```python
from build123d import *

# Parameters (mm, degrees)
SKETCH1_R           = 27
SKETCH1_R_2         = 14
BOSS_EXTRUDE1_DEPTH = 10
SKETCH2_R           = 32.5
BOSS_EXTRUDE2_DEPTH = 2
SKETCH3_W           = 5
SKETCH3_H           = 4.39677325
SKETCH3_W_2         = 4.39677325
SKETCH3_H_2         = 5
BOSS_EXTRUDE3_DEPTH = 10
CUT_EXTRUDE1_REACH  = 49.503
SKETCH4_R           = 0.9
BOSS_EXTRUDE4_DEPTH = 10
BOSS_EXTRUDE5_START = -2
SKETCH6_R           = 14
BOSS_EXTRUDE5_DEPTH = 2


with BuildPart() as part:
    # Sketch1 → Boss-Extrude1 (new body)
    with BuildSketch(Plane(origin=(0, 0, 0), x_dir=(1, 0, 0), z_dir=(0, 1, 0))):
        with Locations(Location((0, 0, 0), (0, 0, 270))):
            Circle(SKETCH1_R)
        with Locations(Location((0, 0, 0), (0, 0, 270))):
            Circle(SKETCH1_R_2, mode=Mode.SUBTRACT)
        with BuildLine():
            Line((-17.5, -17.853571071), (-11.2, -11.426285486))
            ThreePointArc((-11.2, -11.426285486), (0, 16), (11.2, -11.426285486))
            Line((11.2, -11.426285486), (17.5, -17.853571071))
            ThreePointArc((17.5, -17.853571071), (0, 25), (-17.5, -17.853571071))
        make_face(mode=Mode.SUBTRACT)
    extrude(amount=BOSS_EXTRUDE1_DEPTH)

    # Sketch2 → Boss-Extrude2 (add)
    with BuildSketch(Plane.XZ):
        with Locations(Location((0, 0, 0), (0, 0, 270))):
            Circle(SKETCH2_R)
    extrude(amount=BOSS_EXTRUDE2_DEPTH)

    # Sketch3 → Boss-Extrude3 (add)
    with BuildSketch(Plane(origin=(0, 0, 0), x_dir=(1, 0, 0), z_dir=(0, 1, 0))):
        with Locations((0, 27.601613375)):
            Rectangle(SKETCH3_W, SKETCH3_H)
        with Locations((27.601613375, 0)):
            Rectangle(SKETCH3_W_2, SKETCH3_H_2)
        with Locations((0, -27.601613375)):
            Rectangle(SKETCH3_W, SKETCH3_H)
        with Locations((-27.601613375, 0)):
            Rectangle(SKETCH3_W_2, SKETCH3_H_2)
    extrude(amount=BOSS_EXTRUDE3_DEPTH)

    # Sketch4 → Cut-Extrude1 (cut, up to next)
    with BuildSketch(Plane.XZ.offset(2), mode=Mode.PRIVATE) as cut_extrude1_sk1:
        with Locations(Location((0, -7, 0), (0, 0, 270))):
            Circle(SKETCH4_R)
    cut_extrude1_tool1 = extrude(cut_extrude1_sk1.sketch, amount=-CUT_EXTRUDE1_REACH, mode=Mode.PRIVATE) & part.part
    # Sketch4 → Cut-Extrude1 (cut, up to next)
    with BuildSketch(Plane.XZ.offset(2), mode=Mode.PRIVATE) as cut_extrude1_sk2:
        with Locations(Location((-7, 0, 0), (0, 0, 270))):
            Circle(SKETCH4_R)
    cut_extrude1_tool2 = extrude(cut_extrude1_sk2.sketch, amount=-CUT_EXTRUDE1_REACH, mode=Mode.PRIVATE) & part.part
    # Sketch4 → Cut-Extrude1 (cut, up to next)
    with BuildSketch(Plane.XZ.offset(2), mode=Mode.PRIVATE) as cut_extrude1_sk3:
        with Locations(Location((0, 7, 0), (0, 0, 270))):
            Circle(SKETCH4_R)
    cut_extrude1_tool3 = extrude(cut_extrude1_sk3.sketch, amount=-CUT_EXTRUDE1_REACH, mode=Mode.PRIVATE) & part.part
    # Sketch4 → Cut-Extrude1 (cut, up to next)
    with BuildSketch(Plane.XZ.offset(2), mode=Mode.PRIVATE) as cut_extrude1_sk4:
        with Locations(Location((7, 0, 0), (0, 0, 270))):
            Circle(SKETCH4_R)
    cut_extrude1_tool4 = extrude(cut_extrude1_sk4.sketch, amount=-CUT_EXTRUDE1_REACH, mode=Mode.PRIVATE) & part.part
    add(cut_extrude1_tool1.solids().sort_by_distance((0, -2, -7))[0], mode=Mode.SUBTRACT)
    add(cut_extrude1_tool2.solids().sort_by_distance((-7, -2, 0))[0], mode=Mode.SUBTRACT)
    add(cut_extrude1_tool3.solids().sort_by_distance((0, -2, 7))[0], mode=Mode.SUBTRACT)
    add(cut_extrude1_tool4.solids().sort_by_distance((7, -2, 0))[0], mode=Mode.SUBTRACT)

    # Sketch5 → Boss-Extrude4 (add)
    with BuildSketch(Plane(origin=(0, 0, 0), x_dir=(1, 0, 0), z_dir=(0, 1, 0))):
        with BuildLine():
            Line((0, 29.8), (0, 32.5))
            ThreePointArc((0, 32.5), (-32.5, 0), (0, -32.5))
            Line((0, -32.5), (0, -29.8))
            Line((0, -29.8), (-2.5, -29.8))
            Line((-2.5, -29.8), (-2.5, -26.884010118))
            ThreePointArc((-2.5, -26.884010118), (-19.091883092, -19.091883092), (-26.884010118, -2.5))
            Line((-26.884010118, -2.5), (-29.8, -2.5))
            Line((-29.8, -2.5), (-29.8, 2.5))
            Line((-29.8, 2.5), (-26.884010118, 2.5))
            ThreePointArc((-26.884010118, 2.5), (-19.091883092, 19.091883092), (-2.5, 26.884010118))
            Line((-2.5, 26.884010118), (-2.5, 29.8))
            Line((-2.5, 29.8), (0, 29.8))
        make_face()
    extrude(amount=BOSS_EXTRUDE4_DEPTH)

    # Sketch6 → Boss-Extrude5 (add)
    with BuildSketch(Plane(origin=(0, 6.5, 0), x_dir=(1, 0, 0), z_dir=(0, 1, 0)).offset(BOSS_EXTRUDE5_START)):
        with Locations(Location((0, 0, 0), (0, 0, 270))):
            Circle(SKETCH6_R)
    extrude(amount=BOSS_EXTRUDE5_DEPTH)


solid = part.part
```
Geometry: final body of the model. Coordinates: model frame, mm. A direction names the side the tool comes from. Coordinates: 2 decimals unless noted, no trailing zeros. Order: outer loops, then holes, each group sorted by start corner. A loop starts at its lowest first (then second) coordinate and runs counter-clockwise, first axis right, second up. Notation, with made-up numbers: (-18, 44.5) - (12, 44.5) arc R10 ccw to (12, 53.5) - close; hole circle Ø7 at (11.25, 84). An arc over 180 degrees is marked (long way). Return JSON: item names as keys, results as strings. Group by question number.
1. Pull-direction query (Z, two-part tool) for faces 1 (the face through (1, 5, 29.8)), 2 (the face through (-0.345, -1.014, 6.169)), 3 (the face through (29.8, 5, 0)), 4 (the face through (0, 0, 0)); classes: pulls with the +Z half, pulls with the -Z half, needs draft (parallel to the pull), parting line crosses it, or undercut.
2. Cut plane A-A (y = 3.5). Output: boundary loops of the cut face in (x, z), plus the area to 3 significant figures.
3. Set-up query: faces 5 (the face through (-6.11, -1.01, 0.12)), 6 (the face through (0, 5, -31)), 7 (the face through (18.906, 4.93, 19.276)), 8 (the face through (-0.53, 4.93, -15.99)). Return all of +Z, -Z, +X, -X, +Y, -Y with unobstructed straight access to the full face (end or side cutting, diameter ignored); none if empty.
4. Cut plane D-D (z = 13). Output: boundary loops of the cut face in (x, y), plus the area to 3 significant figures.
5. Cut plane C-C (x = 22). Output: boundary loops of the cut face in (y, z), plus the area to 3 significant figures.
6. Material intervals for line 1 along X through (y, z) = (-1.05, 0); line 2 along X through (y, z) = (2.3, 0); line 3 along Y through (x, z) = (-4, 13), sorted ascending. Write a range as [from, to].
7. Pin query (flat end, axial travel): pin 1 (8.5 mm diameter, centred on x = -0.5, z = 3, fed in from +Y); pin 2 (3 mm diameter, centred on y = -0.5, z = -21, fed in from -X); pin 3 (1.5 mm diameter, centred on x = 25.5, y = 7.5, fed in from -Z). Return the tip coordinate at first contact, or that it passes through.
Resolved:
{
 "1": {"face 1": "pulls with the +Z half", "face 2": "undercut", "face 3": "needs draft", "face 4": "undercut"},
 "2": {"outline": "(0, -32.5) - (0, -29.8) - (2.5, -29.8) - (2.5, -26.88) arc R27 ccw to (26.88, -2.5) - (29.8, -2.5) - (29.8, 2.5) - (26.88, 2.5) arc R27 ccw to (2.5, 26.88) - (2.5, 29.8) - (0, 29.8) - (0, 32.5) arc R32.5 ccw to start; hole (-17.5, 17.85) arc R25 ccw (long way) to (17.5, 17.85) - (11.2, 11.43) arc R16 cw (long way) to (-11.2, 11.43) - close; hole circle Ø28 at (0, 0)", "area": "1,340 mm²"},
 "3": {"face 5": "-Y", "face 6": "-Z, +X, +Y", "face 7": "+Z, +X, +Y", "face 8": "+Y"},
 "4": {"outline": "(-29.79, -2) - (29.79, -2) - (29.79, 0) - (23.66, 0) - (23.66, 10) - (21.35, 10) - (21.35, 0) - (12.74, 0) - (12.74, 10) - (5.2, 10) - (5.2, 6.5) - (-5.2, 6.5) - (-5.2, 10) - (-12.74, 10) - (-12.74, 0) - (-21.35, 0) - (-21.35, 10) - (-29.79, 10) - close; hole (-5.2, 0) - (5.2, 0) - (5.2, 4.5) - (-5.2, 4.5) - close", "area": "398 mm²"},
 "5": {"outline": "(-2, -23.92) - (0, -23.92) - (0, -15.65) - (10, -15.65) - (10, -11.87) - (0, -11.87) - (0, 11.87) - (10, 11.87) - (10, 15.65) - (0, 15.65) - (0, 23.92) - (-2, 23.92) - close", "area": "171 mm²"},
 "6": {"line 1": "x = [-32.5, -7.9], [-6.1, 6.1], [7.9, 32.5]", "line 2": "x = [-32.5, -25], [-16, -14], [14, 16], [25, 29.8]", "line 3": "y = [-2, 0], [4.5, 6.5]"},
 "7": {"pin 1": "stops at y = 6.5", "pin 2": "stops at x = -26", "pin 3": "stops at z = -10.79"}
}
